Geometry check sheet. Reference: the model listing, model coordinates, mm. Face numbers are marked on the shaded views. A direction names the side the tool comes from. Give positions to 0.01 mm unless a question says otherwise; leave off trailing zeros. Write each loop counter-clockwise with the first axis right and the second up, starting at its lowest first coordinate (ties: lowest second). Pieces come first, ordered by that corner, then holes.
(1) Cross-section at A-A (z = 14.25). Record the boundary of the cut face in (x, y), and give its area (3 significant figures).
(2) Cross-section at C-C (y = 4.75). Record the boundary of the cut face in (x, z).
(3) Tool access check on the marked faces 1, 2 and 3. Record the directions out of +Z, -Z, +X, -X, +Y, -Y that give a thin tool (end or side, any length) a straight path to the whole face; none if there is none.
(4) Cross-section at D-D (x = 6.5). Record the boundary of the cut face in (y, z).
(5) Cross-section at B-B (z = 3.5). Record the boundary of the cut face in (x, y).
(6) Mould release check, pull along X, two halves, no side actions. Record for the marked faces 4, 5 and 6: +X half, -X half, draft (parallel to the pull), parting line (faces both ways), or undercut.
(7) Depth check by flat-ended pin: P1, Ø5.5, axis at y = -3, z = 12, coming from the -X side; P2, Ø1, axis at y = 4.5, z = 5, coming from the +X side; P3, Ø1.5, axis at x = 8.5, z = 11, coming from the +Y side; P4, Ø1.5, axis at x = -6.5, y = 6.5, coming from the +Z side. Enter the tip coordinate at first touch or a pass-through.
(8) Thickness scan on line 1 along X through (y, z) = (-2, 13.25); line 2 along Y through (x, z) = (9.25, 1.5); line 3 along X through (y, z) = (-2, 9). Record the ranges inside material, lowest first.
```python
from build123d import *

# Parameters (mm, degrees)
SKETCH1_W           = 10
SKETCH1_H           = 18
BOSS_EXTRUDE1_DEPTH = 15
SKETCH3_W           = 5
SKETCH3_H           = 2.3
BOSS_EXTRUDE2_DEPTH = 15
SKETCH4_R           = 3.15
CUT_EXTRUDE1_DEPTH  = 26.475478406
SKETCH6_W           = 2
SKETCH6_H           = 18
CUT_EXTRUDE2_DEPTH  = 8
DRAFT4_ANGLE        = 2


with BuildPart() as part:
    # Sketch1 → Boss-Extrude1 (new body)
    with BuildSketch(Plane.XY):
        Rectangle(SKETCH1_W, SKETCH1_H)
    extrude(amount=BOSS_EXTRUDE1_DEPTH)

    # Sketch3 → Boss-Extrude2 (add)
    with BuildSketch(Plane.XY.offset(15)):
        with Locations((-7.5, -7.85)):
            Rectangle(SKETCH3_W, SKETCH3_H)
        with Locations((7.5, -7.85)):
            Rectangle(SKETCH3_W, SKETCH3_H)
    extrude(amount=-BOSS_EXTRUDE2_DEPTH)

    # Sketch4 → Cut-Extrude1 (cut, through all)
    with BuildSketch(Plane.XZ.offset(9)):
        with Locations(Location((0, 7.5, 0), (0, 0, 270))):
            Circle(SKETCH4_R)
    extrude(amount=-CUT_EXTRUDE1_DEPTH, mode=Mode.SUBTRACT)

    # Sketch6 → Cut-Extrude2 (cut)
    with BuildSketch(Plane.XY.offset(15)):
        Rectangle(SKETCH6_W, SKETCH6_H)
    extrude(amount=-CUT_EXTRUDE2_DEPTH, mode=Mode.SUBTRACT)

    # Draft4
    draft4_faces = [part.faces().sort_by_distance(p)[0] for p in [
        (0, 0, 4.35),
    ]]
    draft(draft4_faces, Plane(origin=(-5, 9, 15), x_dir=(0, 0, 1), z_dir=(0, 1, 0)), DRAFT4_ANGLE)


solid = part.part
```
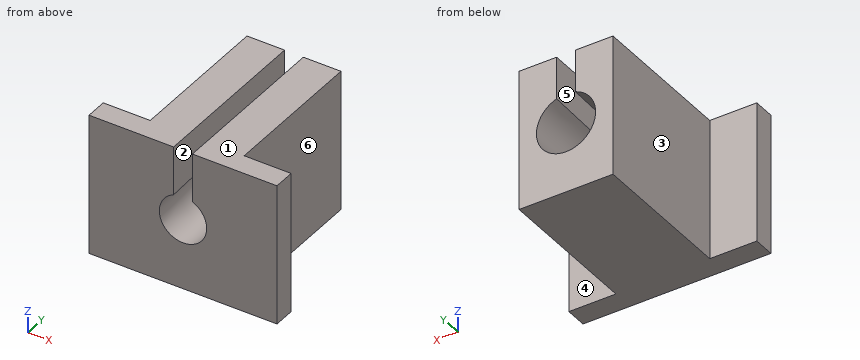
Reply:
1. outline: (-10, -9) - (-1, -9) - (-1, 9) - (-5, 9) - (-5, -6.7) - (-10, -6.7) - close; (1, -9) - (10, -9) - (10, -6.7) - (5, -6.7) - (5, 9) - (1, 9) - close
1. area: 167 mm2
2. outline: (-5, 0) - (5, 0) - (5, 15) - (1, 15) - (1, 10.33) arc R3 cw (long way) to (-1, 10.33) - (-1, 15) - (-5, 15) - close
3. face 1: +Z, +X, -X, +Y, -Y
3. face 2: +Z, +Y, -Y
3. face 3: +Z, -Z, -X, +Y
4. outline: (-9, 0) - (-6.7, 0) - (-6.7, 15) - (-9, 15) - close
5. outline: (-10, -9) - (10, -9) - (10, -6.7) - (5, -6.7) - (5, 9) - (-5, 9) - (-5, -6.7) - (-10, -6.7) - close
6. face 4: draft
6. face 5: undercut
6. face 6: +X half
7. P1: stops at x = -5
7. P2: stops at x = 5
7. P3: stops at y = -6.7
7. P4: passes through
8. line 1: x = -5 to -1, 1 to 5
8. line 2: y = -9 to -6.7
8. line 3: x = -5 to -2.32, 2.32 to 5
